```python
from build123d import *

# Parameters (mm, degrees)
SKETCH2_R           = 2.5
BOSS_EXTRUDE1_DEPTH = 3


with BuildPart() as part:
    # Sketch2 → Boss-Extrude1 (new body)
    with BuildSketch(Plane.XY):
        with BuildLine():
            Line((2.152494721, 5.855657737), (47.152494721, 5.855657737))
            ThreePointArc((47.152494721, 5.855657737), (52.152494721, 0.855657737), (47.152494721, -4.144342263))
            Line((47.152494721, -4.144342263), (2.152494721, -4.144342263))
            ThreePointArc((2.152494721, -4.144342263), (-2.847505279, 0.855657737), (2.152494721, 5.855657737))
        make_face()
        with Locations((8.152494721, 0.855657737)):
            Circle(SKETCH2_R, mode=Mode.SUBTRACT)
        with BuildLine():
            Line((17.152494721, 3.355657737), (47.152494721, 3.355657737))
            ThreePointArc((47.152494721, 3.355657737), (49.652494721, 0.855657737), (47.152494721, -1.644342263))
            Line((47.152494721, -1.644342263), (17.152494721, -1.644342263))
            ThreePointArc((17.152494721, -1.644342263), (14.652494721, 0.855657737), (17.152494721, 3.355657737))
        make_face(mode=Mode.SUBTRACT)
    extrude(amount=BOSS_EXTRUDE1_DEPTH)


solid = part.part
```
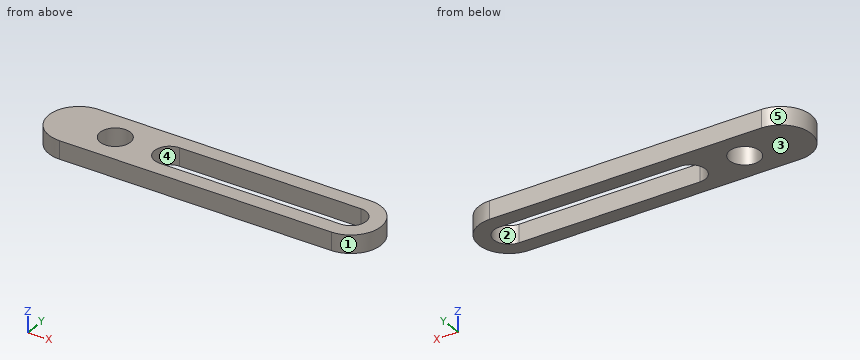
Here's how the part is built. I have some questions about the finished solid (model axes, mm). Face numbers are marked on the shaded views. A direction names the side the tool comes from. Round coordinates to 2 decimals unless told otherwise and drop trailing zeros. Order: outer loops, then holes, each group sorted by start corner. A loop starts at its lowest first (then second) coordinate and runs counter-clockwise, first axis right, second up. Notation, with made-up numbers: M 19,4.25 L 31,4.25 A25 ccw 31,28.25 Z; hole C 11.5,83.25 d2. An arc over 180 degrees is marked long. Answer in a Markdown table with one row per item.
Item 1: If I drill on L1, parallel to X at y = 0.75, z = 0.65; L2, parallel to Y at x = 30, z = 1.7; L3, parallel to X at y = 0.5, z = 0.2, over which ranges is the centre line in solid material (lowest first)? Write a range as from..to.
A:
| item | result |
|---|---|
| L1 | x = -2.85..5.65, 10.65..14.65, 49.65..52.15 |
| L2 | y = -4.14..-1.64, 3.36..5.86 |
| L3 | x = -2.83..5.68, 10.63..14.68, 49.63..52.14 |
Item 2: Imagine slicing it at D-D, the plane y = 2.75. Write out the boundary of the cut face in (x, z).
A:
| item | result |
|---|---|
| outline | M -2.47,0 L 6.52,0 L 6.52,3 L -2.47,3 Z; M 9.78,0 L 15.52,0 L 15.52,3 L 9.78,3 Z; M 48.78,0 L 51.78,0 L 51.78,3 L 48.78,3 Z |
Item 3: Imagine slicing it at C-C, the plane z = 1.65. Write out the boundary of the cut face in (x, y).
A:
| item | result |
|---|---|
| outline | M 2.15,-4.14 L 47.15,-4.14 A5 ccw 47.15,5.86 L 2.15,5.86 A5 ccw Z; hole C 8.15,0.86 d5; hole M 17.15,-1.64 L 47.15,-1.64 A2.5 ccw 47.15,3.36 L 17.15,3.36 A2.5 ccw Z |
Item 4: Imagine slicing it at A-A, the plane x = 43. Write out the boundary of the cut face in (y, z).
A:
| item | result |
|---|---|
| outline | M -4.14,0 L -1.64,0 L -1.64,3 L -4.14,3 Z; M 3.36,0 L 5.86,0 L 5.86,3 L 3.36,3 Z |
Item 5: Thinking about a two-plate mould opening in X: for the marked faces 3, 4 and 5, which applies, +X half, -X half, draft (parallel to the pull), parting line (faces both ways), or undercut?
A:
| item | result |
|---|---|
| face 3 | draft |
| face 4 | undercut |
| face 5 | -X half |
Item 6: For the marked faces 1 and 2, which set-ups out of +Z, -Z, +X, -X, +Y, -Y let a thin tool reach every point of the face, with its end or its side?
A:
| item | result |
|---|---|
| face 1 | +Z, -Z, +X |
| face 2 | +Z, -Z |
Item 7: I'm going to push flat-ended pins straight in: pin 1 (3 mm diameter, centred on x = 40.5, y = 0, fed in from +Z); pin 2 (3 mm diameter, centred on x = 44.5, y = 2.5, fed in from -Z); pin 3 (1.5 mm diameter, centred on y = 4, z = 2, fed in from +X). Where does each tip first touch, or does it pass through?
A:
| item | result |
|---|---|
| pin 1 | passes through |
| pin 2 | stops at z = 0 |
| pin 3 | stops at x = 51.54 |
Item 8: Imagine slicing it at B-B, the plane y = -1. Write out the boundary of the cut face in (x, z), and give its area (3 significant figures).
A:
| item | result |
|---|---|
| outline | M -2.49,0 L 6.48,0 L 6.48,3 L -2.49,3 Z; M 9.83,0 L 15.48,0 L 15.48,3 L 9.83,3 Z; M 48.83,0 L 51.8,0 L 51.8,3 L 48.83,3 Z |
| area | 52.8 mm2 |
